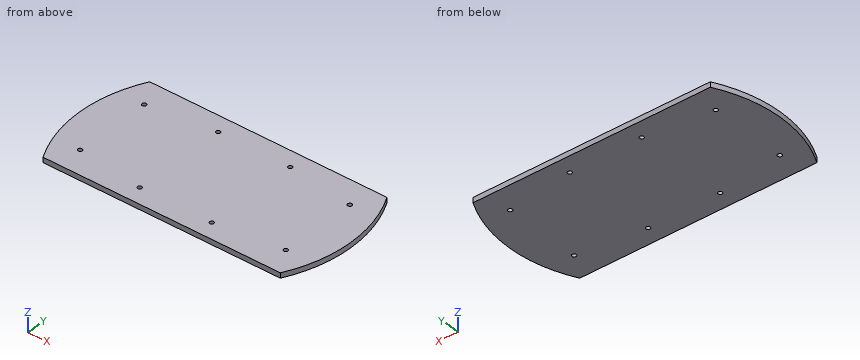
Autodesk Fusion 360 part; units mm, degrees
sketch "Sketch1" plane through (0, 0, 0) normal (0, 0, 1) x (1, 0, 0)
  circle A0 centre (-80, -30) radius 1.65
  line L0 (0, 2.5) -> (0, 20)
  line L1 (20, 0) -> (2.5, 0)
  circle A1 centre (-80, 30) radius 1.65
  circle A2 centre (80, -30) radius 1.65
  circle A3 centre (80, 30) radius 1.65
  line L2 (-28, 36.75) -> (28, 36.75) construction
  line L3 (28, 36.75) -> (28, -36.75) construction
  line L4 (28, -36.75) -> (-28, -36.75) construction
  line L5 (-28, -36.75) -> (-28, 36.75) construction
  circle A4 centre (-28, 36.75) radius 1.6
  circle A5 centre (28, 36.75) radius 1.6
  circle A6 centre (-28, -36.75) radius 1.6
  circle A7 centre (28, -36.75) radius 1.6
  line L6 (-92.3309, -50) -> (92.3309, -50)
  line L7 (-92.3309, 50) -> (92.3309, 50)
  arc A8 (-92.3309, 50) -> (-92.3309, -50) centre (0, 0) ccw
  arc A9 (92.3309, -50) -> (92.3309, 50) centre (0, 0) ccw
  dimension "d1" = 210
  dimension "d2" = 3.3
  dimension "d3" = 80
  dimension "d4" = 30
  dimension "d5" = 56
  dimension "d6" = 73.5
  dimension "d7" = 3.2
  dimension "d8" = 3.2
  dimension "d9" = 3.2
  dimension "d10" = 3.2
  dimension "d11" = 50
extrude "Extrude1" add sketch "Sketch1" along normal blind 4
equation "d6 = 28 mm + 45.5 mm"
Source: CAD feature listing. Evaluate the final solid. Frame: model axes, mm. Coordinates: 2 decimals unless noted, no trailing zeros. Return JSON: item names as keys, results as strings. Group by question number.
1) Contact query for a flat-ended pin moving along its axis: P1, Ø2, axis at y = -29, z = 1, coming from the +X side. Output: stop coordinate, or through.
2) Ray query, line 1 along Y through (x, z) = (-80, 2.2); line 2 along Y through (x, z) = (-28, 1.2); line 3 along X through (y, z) = (6.5, 3.5). Return the intervals inside material, ascending.
3) Section query A-A, the plane z = 1.4. State how many separate pieces and enclosed holes the cut face has, plus the area to 3 significant figures.
From the geometry:
{
 "1": {"P1": "x = 101.2"},
 "2": {"line 1": "-50 to -31.65, -28.35 to 28.35, 31.65 to 50", "line 2": "-50 to -38.35, -35.15 to 35.15, 38.35 to 50", "line 3": "-104.8 to 104.8"},
 "3": {"separate pieces": "1", "enclosed holes": "8", "area": "20,100 mm²"}
}
